```python
from build123d import *

# Parameters (mm, degrees)
SKETCH1_R           = 37.5
SKETCH1_R_2         = 28.5
BOSS_EXTRUDE1_DEPTH = 3
BOSS_EXTRUDE2_START = -3
BOSS_EXTRUDE2_DEPTH = 3
SKETCH6_R           = 1.65
CUT_EXTRUDE2_DEPTH  = 10
SKETCH7_R           = 3.1
CUT_EXTRUDE3_DEPTH  = 1.5
FILLET1_R           = 3


with BuildPart() as part:
    # Sketch1 → Boss-Extrude1 (new body)
    with BuildSketch(Plane(origin=(0, 0, 0), x_dir=(1, 0, 0), z_dir=(0, 1, 0))):
        with Locations(Location((0, 0, 0), (0, 0, 270))):
            Circle(SKETCH1_R)
        with Locations(Location((0, 0, 0), (0, 0, 270))):
            Circle(SKETCH1_R_2, mode=Mode.SUBTRACT)
    extrude(amount=BOSS_EXTRUDE1_DEPTH)

    # Sketch3 → Boss-Extrude2 (add)
    with BuildSketch(Plane(origin=(0, 3, 0), x_dir=(1, 0, 0), z_dir=(0, 1, 0)).offset(BOSS_EXTRUDE2_START)):
        with BuildLine():
            ThreePointArc((37.135052578, 5.218991286), (45.901049183, 0), (37.135052578, -5.218991286))
            ThreePointArc((37.135052578, -5.218991286), (37.5, 0), (37.135052578, 5.218991286))
        make_face()
        with BuildLine():
            ThreePointArc((-14.047747253, -34.769394546), (-22.950524592, -39.751474653), (-23.087305325, -29.55040326))
            ThreePointArc((-23.087305325, -29.55040326), (-18.75, -32.475952642), (-14.047747253, -34.769394546))
        make_face()
        with BuildLine():
            ThreePointArc((-23.087305325, 29.55040326), (-22.950524592, 39.751474653), (-14.047747253, 34.769394546))
            ThreePointArc((-14.047747253, 34.769394546), (-18.75, 32.475952642), (-23.087305325, 29.55040326))
        make_face()
    extrude(amount=BOSS_EXTRUDE2_DEPTH)

    # Sketch6 → Cut-Extrude2 (cut)
    with BuildSketch(Plane(origin=(0, 3, 0), x_dir=(1, 0, 0), z_dir=(0, 1, 0))):
        with Locations(Location((41, 0, 0), (0, 0, 270))):
            Circle(SKETCH6_R)
        with Locations(Location((-20.5, -35.507041555, 0), (0, 0, 270))):
            Circle(SKETCH6_R)
        with Locations(Location((-20.5, 35.507041555, 0), (0, 0, 270))):
            Circle(SKETCH6_R)
    extrude(amount=-CUT_EXTRUDE2_DEPTH, mode=Mode.SUBTRACT)

    # Sketch7 → Cut-Extrude3 (cut)
    with BuildSketch(Plane(origin=(0, 3, 0), x_dir=(1, 0, 0), z_dir=(0, 1, 0))):
        with Locations(Location((41, 0, 0), (0, 0, 270))):
            Circle(SKETCH7_R)
        with Locations(Location((-20.5, -35.507041555, 0), (0, 0, 270))):
            Circle(SKETCH7_R)
        with Locations(Location((-20.5, 35.507041555, 0), (0, 0, 270))):
            Circle(SKETCH7_R)
    extrude(amount=-CUT_EXTRUDE3_DEPTH, mode=Mode.SUBTRACT)

    # Fillet1
    fillet1_edges = [part.edges().sort_by_distance(p)[0] for p in [
        (37.135052578, 1.5, 5.218991286),
        (37.135052578, 1.5, -5.218991286),
        (-23.087305325, 1.5, 29.55040326),
        (-14.047747253, 1.5, 34.769394546),
        (-14.047747253, 1.5, -34.769394546),
        (-23.087305325, 1.5, -29.55040326),
    ]]
    fillet(fillet1_edges, radius=FILLET1_R)


solid = part.part
```
Check sheet for the modelled part. Datum: model origin and axes. Units: mm. A direction names the side the tool comes from. Coordinates: 2 decimals unless noted, no trailing zeros. Loops run counter-clockwise (first coordinate to the right, second up) from the corner with the lowest first, then second, coordinate; pieces in that order, holes last.
1) Material ranges on probe 1 along Z at (x, y) = (-19, 1); probe 2 along Z at (x, y) = (-21, 1.1); probe 3 along Z at (x, y) = (-1, 1.8), recorded low to high.
2) Sectioned sample at C-C (z = 22.5). Record the boundary of the cut face in (x, y), and give its area (3 significant figures).
3) Gauge pin test, flat ends, axial feed: pin 1 (3 mm diameter, centred on x = 40.5, z = -1, fed in from +Y); pin 2 (1 mm diameter, centred on x = -9.5, y = 1, fed in from -Z); pin 3 (1.5 mm diameter, centred on x = 14, y = 2.5, fed in from -Z). Record the tip position at first contact, or that the pin passes through.
4) Access from +Z, -Z, +X, -X, +Y, -Y to the whole of each face (thin tool, end or side, straight path). Record for faces 5 (the face through (-20.364, 2.26, -38.604)), 6 (the face through (42.39, 0.76, 0.89)).
5) Sectioned sample at A-A (z = 0). Record the boundary of the cut face in (x, y), and give its area (3 significant figures).
6) Sectioned sample at D-D (y = 0.6). Count the separate pieces of the cut face and the enclosed holes in it, and give its area (3 significant figures).
7) Sectioned sample at B-B (x = 7.5). Record the boundary of the cut face in (y, z), and give its area (3 significant figures).
8) Release check for a two-part mould opening along Z. For faces 1 (the face through (19.12, 1.48, -32.26)), 2 (the face through (18.374, 1.479, 32.69)), 3 (the face through (-27.82, 1.48, -6.18)), 4 (the face through (45.9, 1.5, -0.1)) record: released by +Z, released by -Z, zero draft, split by the parting line, or undercut.
Check sheet entries:
1. probe 1: z = -40.47 to -36.19, -34.82 to -21.24, 21.24 to 34.82, 36.19 to 40.47
1. probe 2: z = -40.46 to -37.08, -33.93 to -19.27, 19.27 to 33.93, 37.08 to 40.46
1. probe 3: z = -37.49 to -28.48, 28.48 to 37.49
2. outline: (-30, 0) - (-17.49, 0) - (-17.49, 3) - (-30, 3) - close; (17.49, 0) - (30, 0) - (30, 3) - (17.49, 3) - close
2. area: 75.0 mm2
3. pin 1: stops at y = 1.5
3. pin 2: stops at z = -36.4
3. pin 3: stops at z = -35.08
4. face 5: +Y
4. face 6: +Y, -Y
5. outline: (-37.5, 0) - (-28.5, 0) - (-28.5, 3) - (-37.5, 3) - close; (28.5, 0) - (39.35, 0) - (39.35, 1.5) - (37.9, 1.5) - (37.9, 3) - (28.5, 3) - close; (42.65, 0) - (45.9, 0) - (45.9, 3) - (44.1, 3) - (44.1, 1.5) - (42.65, 1.5) - close
5. area: 65.0 mm2
6. separate pieces: 1
6. enclosed holes: 4
6. area: 2,110 mm2
7. outline: (0, -36.74) - (3, -36.74) - (3, -27.5) - (0, -27.5) - close; (0, 27.5) - (3, 27.5) - (3, 36.74) - (0, 36.74) - close
7. area: 55.5 mm2
8. face 1: released by -Z
8. face 2: released by +Z
8. face 3: undercut
8. face 4: split by the parting line
